from build123d import *

# Parameters (mm, degrees)
SKETCH1_W              = 1.3
SKETCH1_H              = 8
BASE_SHAPE_DEPTH       = 2.9
SKETCH2_R              = 5
FORWARD_CUT_TEMP_DEPTH = 1
FILLET1_R              = 1
CUT_EXTRUDE1_REACH     = 4.9
SKETCH4_W              = 61.6
SKETCH4_H              = 20


with BuildPart() as part:
    # Sketch1 → Base shape (new body)
    with BuildSketch(Plane.XY):
        Polygon((39.5, 10), (-39.5, 10), (-39.5, 6), (-36.5, 6), (-36.5, 7.5), (-34.3, 7.5), (-34.3, 2.5), (-36.5, 2.5), (-36.5, 4), (-39.5, 4), (-39.5, -4), (-36.5, -4), (-36.5, -2.5), (-34.3, -2.5), (-34.3, -7.5), (-36.5, -7.5), (-36.5, -6), (-39.5, -6), (-39.5, -10), (39.5, -10), (39.5, -6), (36.5, -6), (36.5, -7.5), (34.3, -7.5), (34.3, -2.5), (36.5, -2.5), (36.5, -4), (39.5, -4), (39.5, 4), (36.5, 4), (36.5, 2.5), (34.3, 2.5), (34.3, 7.5), (36.5, 7.5), (36.5, 6), (39.5, 6), align=None)
        with Locations((-40.15, 0)):
            Rectangle(SKETCH1_W, SKETCH1_H)
        with Locations((40.15, 0)):
            Rectangle(SKETCH1_W, SKETCH1_H)
    extrude(amount=BASE_SHAPE_DEPTH)

    # Sketch2 → Forward cut _temp (cut)
    with BuildSketch(Plane.XY.offset(2.9)):
        Circle(SKETCH2_R)
    extrude(amount=-FORWARD_CUT_TEMP_DEPTH, mode=Mode.SUBTRACT)

    # Fillet1
    fillet1_edges = [part.edges().sort_by_distance(p)[0] for p in [
        (36.5, -2.5, 1.45),
        (34.3, -2.5, 1.45),
        (34.3, -7.5, 1.45),
        (36.5, -7.5, 1.45),
        (-36.5, -7.5, 1.45),
        (-34.3, -7.5, 1.45),
        (-34.3, -2.5, 1.45),
        (-36.5, -2.5, 1.45),
        (-36.5, 2.5, 1.45),
        (-34.3, 2.5, 1.45),
        (-34.3, 7.5, 1.45),
        (-36.5, 7.5, 1.45),
        (36.5, 7.5, 1.45),
        (34.3, 7.5, 1.45),
        (34.3, 2.5, 1.45),
        (36.5, 2.5, 1.45),
    ]]
    fillet(fillet1_edges, radius=FILLET1_R)

    # Sketch4 → Cut-Extrude1 (cut, up to next)
    with BuildSketch(Plane.XY.offset(2.9), mode=Mode.PRIVATE) as cut_extrude1_sk1:
        with Locations((-10, 0)):
            Rectangle(SKETCH4_W, SKETCH4_H)
    cut_extrude1_tool1 = extrude(cut_extrude1_sk1.sketch, amount=-CUT_EXTRUDE1_REACH, mode=Mode.PRIVATE) & part.part
    add(cut_extrude1_tool1.solids().sort_by_distance((-10, 0, 2.9))[0], mode=Mode.SUBTRACT)


solid = part.part
For this review, take the finished solid that the model builds, in its own axes (mm). A direction names the side the tool comes from. Coordinates: 2 decimals unless noted, no trailing zeros. Loops run counter-clockwise (first coordinate to the right, second up) from the corner with the lowest first, then second, coordinate; pieces in that order, holes last. Notation, with made-up numbers: (24.25, 56) - (42.25, 56) arc R17 cw to (42.25, 79) - close; hole circle Ø11 at (8, -36.5). An arc over 180 degrees is marked (long way). Return JSON: item names as keys, results as strings.
Item 1: Insertion check: pin 1 (0.9 mm diameter, centred on y = -8.5, z = 1.5, fed in from +X); pin 2 (0.9 mm diameter, centred on y = -5, z = 2, fed in from +X); pin 3 (1.5 mm diameter, centred on x = 28, y = 0, fed in from -Z). Each pin has a flat end and moves straight along its axis. Give the tip position at first contact, or say it passes through.
Determined:
{"pin 1": "stops at x = 39.5", "pin 2": "stops at x = 34.3", "pin 3": "stops at z = 0"}
Item 2: Take a section at B-B (z = 0.5). Give the boundary of the cut face in (x, y), then the cut area to 3 significant figures.
Determined:
{"outline": "(20.8, -10) - (39.5, -10) - (39.5, -6) - (36.5, -6) - (36.5, -6.5) arc R1 cw to (35.5, -7.5) - (35.3, -7.5) arc R1 cw to (34.3, -6.5) - (34.3, -3.5) arc R1 cw to (35.3, -2.5) - (35.5, -2.5) arc R1 cw to (36.5, -3.5) - (36.5, -4) - (40.8, -4) - (40.8, 4) - (36.5, 4) - (36.5, 3.5) arc R1 cw to (35.5, 2.5) - (35.3, 2.5) arc R1 cw to (34.3, 3.5) - (34.3, 6.5) arc R1 cw to (35.3, 7.5) - (35.5, 7.5) arc R1 cw to (36.5, 6.5) - (36.5, 6) - (39.5, 6) - (39.5, 10) - (20.8, 10) - close", "area": "352 mm2"}
Item 3: For faces 1 (the flat face through (39.5, -8, 1)), 2 (the flat face through (40.8, 0, 1)), 3 (the cylindrical face through (36.199, 7.215, 1.47)), 4 (the flat face through (38, 6, 1)), 5 (the flat face through (30, -10, 1)), list the 3-axis set-ups (+Z, -Z, +X, -X, +Y, -Y) from which the entire face can be reached by the end or side of a thin tool; tool diameter is ignored.
Determined:
{"face 1": "+Z, -Z, +X, -Y", "face 2": "+Z, -Z, +X, +Y, -Y", "face 3": "+Z, -Z", "face 4": "+Z, -Z, +X", "face 5": "+Z, -Z, +X, -X, -Y"}
Item 4: Take a section at A-A (x = 37). Give the boundary of the cut face in (y, z).
Determined:
{"outline": "(-10, 0) - (-6, 0) - (-6, 2.9) - (-10, 2.9) - close; (-4, 0) - (4, 0) - (4, 2.9) - (-4, 2.9) - close; (6, 0) - (10, 0) - (10, 2.9) - (6, 2.9) - close"}
Item 5: Mouldability with a two-part tool opening along X and no side actions: class faces 6 (the flat face through (30, 10, 1)), 7 (the flat face through (20.8, 0, 1)), 8 (the cylindrical face through (34.601, 2.785, 1.47)), 9 (the flat face through (39.5, 8, 1)) as pulls with the +X half, pulls with the -X half, needs draft (parallel to the pull), parting line crosses it, or undercut.
Determined:
{"face 6": "needs draft", "face 7": "pulls with the -X half", "face 8": "undercut", "face 9": "pulls with the +X half"}
Item 6: Take a section at D-D (y = 8). Give the boundary of the cut face in (x, z).
Determined:
{"outline": "(20.8, 0) - (39.5, 0) - (39.5, 2.9) - (20.8, 2.9) - close"}
Item 7: Take a section at C-C (y = -3). Give the boundary of the cut face in (x, z).
Determined:
{"outline": "(20.8, 0) - (34.43, 0) - (34.43, 2.9) - (20.8, 2.9) - close; (36.37, 0) - (40.8, 0) - (40.8, 2.9) - (36.37, 2.9) - close"}
Item 8: For line 1 (Y direction, x = 38, z = 2.6); line 2 (Y direction, x = 35.25, z = 2.75); line 3 (X direction, y = -4.5, z = 1.85), list the stretches that pass through material, from the lowest coordinate up.
Determined:
{"line 1": "y = -10 to -6, -4 to 4, 6 to 10", "line 2": "y = -10 to -7.5, -2.5 to 2.5, 7.5 to 10", "line 3": "x = 20.8 to 34.3"}
